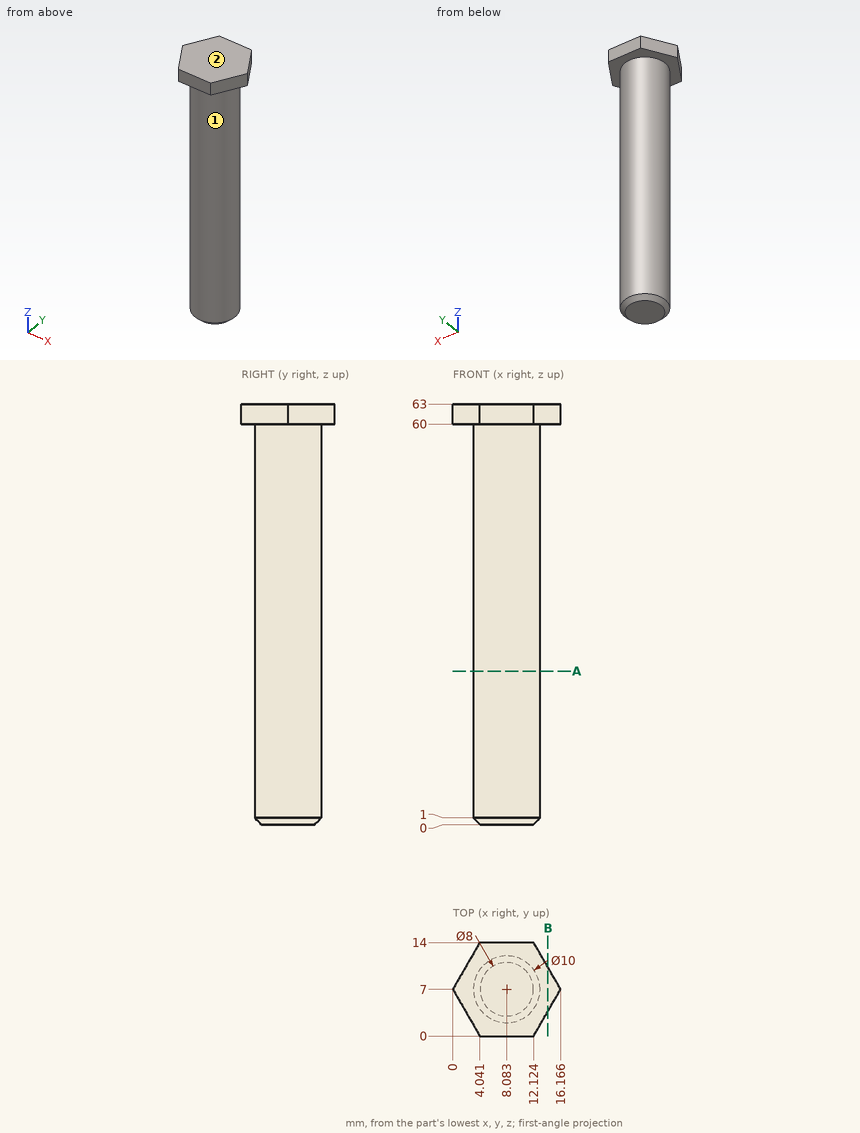
Drawing for the job (mm, zero at the part's lowest x, y, z). A direction names the side the tool comes from. Round coordinates to 2 decimals unless told otherwise and drop trailing zeros. Loops run counter-clockwise (first coordinate to the right, second up) from the corner with the lowest first, then second, coordinate; pieces in that order, holes last. Notation, with made-up numbers: M 88.25,-14 L 113.25,-14 A16 ccw 113.25,2 Z; hole C -4,42 d8. An arc over 180 degrees is marked long. Use a Markdown table: item, result. Add a question column.
(1) Which spindle directions (+Z, -Z, +X, -X, +Y, -Y) get a long thin tool onto all of the face, cutting with end or side? Do the marked faces 1 and 2. Say none if no direction does.
(2) Drill centre lines: line 1 (X direction, y = 4, z = 35.5) (1 decimal); line 2 (Z direction, x = 6.5, y = 12); line 3 (X direction, y = 6.75, z = 42). Where is each one in solid material? Low to high.
(3) Flat gauge pins, fed straight in: pin 1 (5 mm diameter, centred on x = 3.5, z = 41.5, fed in from -Y) (1 decimal); pin 2 (4 mm diameter, centred on y = 12.5, z = 12.5, fed in from -X); pin 3 (3 mm diameter, centred on x = 10, z = 7, fed in from -Y). Where does each tip first touch, or does it go through?
(4) Cut at A-A (z = 23). Give the cut face in (x, y).
(5) Cut at B-B (x = 14.25). Give the cut face in (y, z), and give its area (3 significant figures).
Geometry says:
| question | item | result |
|---|---|---|
| 1 | face 1 | -Z |
| 1 | face 2 | +Z, +X, -X, +Y, -Y |
| 2 | line 1 | x = 4.1 to 12.1 |
| 2 | line 2 | z = 60 to 63 |
| 2 | line 3 | x = 3.09 to 13.08 |
| 3 | pin 1 | stops at y = 2.5 |
| 3 | pin 2 | stops at x = 4.51 |
| 3 | pin 3 | stops at y = 2.02 |
| 4 | outline | C 8.08,7 d10 |
| 5 | outline | M 3.68,60 L 10.32,60 L 10.32,63 L 3.68,63 Z |
| 5 | area | 19.9 mm² |
